Here's how the part is built. I have some questions about the finished solid (model axes, mm). A direction names the side the tool comes from. Round coordinates to 2 decimals unless told otherwise and drop trailing zeros. Order: outer loops, then holes, each group sorted by start corner. A loop starts at its lowest first (then second) coordinate and runs counter-clockwise, first axis right, second up. Notation, with made-up numbers: (79, 67) - (89, 67) arc R21 ccw to (89, 99) - close; hole circle Ø5 at (-2, 14). An arc over 180 degrees is marked (long way). Answer as a JSON object with one key per item and string values.
```python
from build123d import *
from build123d.topology import SkipClean

# Parameters (mm, degrees)
EXTRUDE_1_DEPTH          = 9.5
CUT_EXTRUDE_1_DEPTH      = 19.754173631
CUT_EXTRUDE_1_DEPTH_BACK = 19.754173631
SKETCH_3_R               = 6
CUT_EXTRUDE_3_DEPTH      = 18.322626143
CUT_EXTRUDE_3_DEPTH_BACK = 18.322626143
SKETCH_5_R               = 6.5
CUT_EXTRUDE_4_DEPTH      = 6.5
EXTRUDE_2_DEPTH          = 6.5
EXTRUDE_START            = -2.479634576
EXTRUDE_3_DEPTH          = 3.479634576
CUT_EXTRUDE_5_DEPTH      = 21.256440541
CUT_EXTRUDE_5_DEPTH_BACK = 21.256440541
SKETCH_10_R              = 5
FILLET_1_R               = 6


with BuildPart() as part:
    # Sketch 2 → Extrude 1 (new, symmetric)
    with BuildSketch(Plane.XY):
        with BuildLine():
            Line((3.046153846, 5.169230769), (-6, 10.5))
            Line((-6, 10.5), (-14.485281374, 10.5))
            Line((-14.485281374, 10.5), (-14.485281374, -6))
            Line((-14.485281374, -6), (0, -6))
            ThreePointArc((0, -6), (5.788582927, -1.578704435), (3.046153846, 5.169230769))
        make_face()
    extrude(amount=EXTRUDE_1_DEPTH, both=True)

    # Sketch 3 → Cut-Extrude 1 (cut, two sides: drawn at the far end of the back side and taken through both)
    with BuildSketch(Plane(origin=(-3.249999973, 5.629165078, 0), x_dir=(0.8660254037844386, 0.4999999999999999, 0), z_dir=(-0.49999999999999994, 0.8660254037844387, 0)).offset(-CUT_EXTRUDE_1_DEPTH_BACK)):
        Circle(SKETCH_3_R)
        with BuildLine():
            ThreePointArc((6, 0), (3.333421398, -4.988817674), (-2.296100594, -5.543277195))
            Line((-2.296100594, -5.543277195), (6, -8.979634576))
            Line((6, -8.979634576), (6, 0))
        make_face()
        with BuildLine():
            Line((6, 8.979634576), (-2.296100594, 5.543277195))
            ThreePointArc((-2.296100594, 5.543277195), (3.333421398, 4.988817674), (6, 0))
            Line((6, 0), (6, 8.979634576))
        make_face()
    extrude(amount=CUT_EXTRUDE_1_DEPTH + CUT_EXTRUDE_1_DEPTH_BACK, mode=Mode.SUBTRACT)

    # Sketch 4 → Cut-Extrude 3 (cut, two sides: drawn at the far end of the back side and taken through both)
    with BuildSketch(Plane(origin=(-4.242640687, 4.242640687, 0), x_dir=(-0.7071067811865511, 0.707106781186544, 0), z_dir=(-0.707106781186544, -0.7071067811865511, 0)).offset(-CUT_EXTRUDE_3_DEPTH_BACK)):
        with BuildLine():
            Line((-12, -6.5), (-4, -6.5))
            add(Edge.make_bspline(
                [(-4, -6.5), (0, -6.5), (0, -2)],
                knots=[0, 0, 0, 1.570796327, 1.570796327, 1.570796327], degree=2, weights=[1, 0.707106781, 1]))
            Line((0, -2), (0, 2))
            add(Edge.make_bspline(
                [(0, 2), (0, 6.5), (-4, 6.5)],
                knots=[4.71238898, 4.71238898, 4.71238898, 6.283185307, 6.283185307, 6.283185307], degree=2, weights=[1, 0.707106781, 1]))
            Line((-4, 6.5), (-12, 6.5))
            Line((-12, 6.5), (-12, -6.5))
        make_face()
    extrude(amount=CUT_EXTRUDE_3_DEPTH + CUT_EXTRUDE_3_DEPTH_BACK, mode=Mode.SUBTRACT)

    # Sketch 5 → Cut-Extrude 4 (cut, symmetric)
    with BuildSketch(Plane.XY):
        Circle(SKETCH_5_R)
    extrude(amount=CUT_EXTRUDE_4_DEPTH, both=True, mode=Mode.SUBTRACT)

    # Sketch 6 → Extrude 2 (add, symmetric)
    with BuildSketch(Plane.XY):
        with BuildLine():
            Line((-6.502520338, 3.75132157), (-8.445640507, 2.629460617))
            Line((-8.445640507, 2.629460617), (-8.980852778, -0.495571404))
            ThreePointArc((-8.980852778, -0.495571404), (-7.713770339, 0.615313333), (-6.312263919, 1.550910769))
            ThreePointArc((-6.312263919, 1.550910769), (-6.076847823, 2.306928809), (-5.751252167, 3.028712353))
            ThreePointArc((-5.751252167, 3.028712353), (-5.855186593, 3.672492332), (-6.502520338, 3.75132157))
        make_face()
    extrude(amount=EXTRUDE_2_DEPTH, both=True)

    # Extrude 3: read off the stored shape, not the designer's step
    # Extrude 3 outline → Extrude 3 (add)
    with BuildSketch(Plane(origin=(0, 0, 6.5), x_dir=(-1, 0, 0), z_dir=(0, 0, -1)).offset(EXTRUDE_START)):
        with BuildLine():
            Line((4.242640687, -4.242640687), (10.137783082, 1.652501708))
            Line((10.137783082, 1.652501708), (3.25, 5.629165125))
            add(Edge.make_bspline(
                [(3.25, 5.629165125), (2.607695155, 6), (0, 6)],
                knots=[0, 0, 0, 1, 1, 1], degree=2))
            ThreePointArc((0, 6), (-5.543277195, -2.296100594), (4.242640687, -4.242640687))
        make_face()
    extrude_3 = extrude(amount=EXTRUDE_3_DEPTH)

    # Mirror 1: Extrude 3 across plane
    with SkipClean():  # the faces are left unmerged after this step: merging them gives an invalid solid
        add(extrude_3.mirror(Plane.XY))

    # Sketch 10 → Cut-Extrude 5 (cut, two sides: drawn at the far end of the back side and taken through both)
    with SkipClean():  # the faces are left unmerged after this step: merging them gives an invalid solid
        with BuildSketch(Plane.XY.offset(-CUT_EXTRUDE_5_DEPTH_BACK)):
            Circle(SKETCH_10_R)
        extrude(amount=CUT_EXTRUDE_5_DEPTH + CUT_EXTRUDE_5_DEPTH_BACK, mode=Mode.SUBTRACT)

    # Fillet 1
    fillet_1_edges = [part.edges().sort_by_distance(p)[0] for p in [
        (-6, 10.5, -8.008328799),
        (-6, 10.5, 8.008328799),
    ]]
    fillet(fillet_1_edges, radius=FILLET_1_R)


solid = part.part
```
1. If I drill on L1, parallel to X at y = 0, z = -7.95; L2, parallel to Y at x = 0, z = -6.55; L3, parallel to Z at x = -2.5, y = 7.5, over which ranges is the centre line in solid material (lowest first)? Write a range as [from, to].
Responses:
{"L1": "[-14.49, -5], [5, 6]", "L2": "[-6, -5], [5, 6]", "L3": "[-9.5, -7.15], [7.15, 9.5]"}
2. Imagine slicing it at A-A (x = 0.75). List the corners of the cut face in (y, z) for me, plus the area to 3 significant figures.
Responses:
{"outline": "(-5.95, -9.5) - (-4.94, -9.5) - (-4.94, -5.5) - (-5.95, -5.5) - close; (-5.95, 5.5) - (-4.94, 5.5) - (-4.94, 9.5) - (-5.95, 9.5) - close; (4.94, -9.5) - (6.52, -9.5) - (6.52, -8.11) - (5.95, -8) - (5.95, -5.5) - (4.94, -5.5) - close; (4.94, 5.5) - (5.95, 5.5) - (5.95, 8) - (6.52, 8.11) - (6.52, 9.5) - (4.94, 9.5) - close", "area": "17.8 mm2"}
3. For faces 1 (the face through (-5.85, 3.67, 0.07)), 2 (the face through (-11.695, -3.209, 0.028)), 3 (the face through (-3.84, 5.29, -5.78)), which set-ups out of +Z, -Z, +X, -X, +Y, -Y let a thin tool reach every point of the face, with its end or its side?
Responses:
{"face 1": "none", "face 2": "+X, -Y", "face 3": "+Y"}
4. Imagine slicing it at C-C (x = -2.5). Give the number of separate pieces and of enclosed holes in the cut face, plus the area to 3 significant figures.
Responses:
{"separate pieces": "4", "enclosed holes": "0", "area": "37.0 mm2"}
5. For P1, Ø3, axis at y = -3, z = -1.5, coming from the +X side, with a flat end and sliding along its axis, tell me the tip position at first contact or that it passes through.
Responses:
{"P1": "x = -9.99"}
6. Imagine slicing it at B-B (z = -1). List the corners of the cut face in (x, y) for me, plus the area to 3 significant figures.
Responses:
{"outline": "(-14.49, -6) - (-8.98, -0.5) arc R12.85 cw to (-6.31, 1.55) arc R6.5 cw to (-5.75, 3.03) arc R0.54 ccw to (-6.5, 3.75) - (-8.37, 2.67) - (-12.89, 10.5) - (-14.49, 10.5) - close", "area": "70.2 mm2"}
7. Thinking about a two-plate mould opening in Z: for faces 4 (the face through (-5.462, -3.024, 6.007)), 5 (the face through (-9, 2, 9.5)), 6 (the face through (-1.08, -4.88, 7.47)), which applies, pulls with the +Z half, pulls with the -Z half, needs draft (parallel to the pull), parting line crosses it, or undercut?
Responses:
{"face 4": "undercut", "face 5": "pulls with the +Z half", "face 6": "needs draft"}
